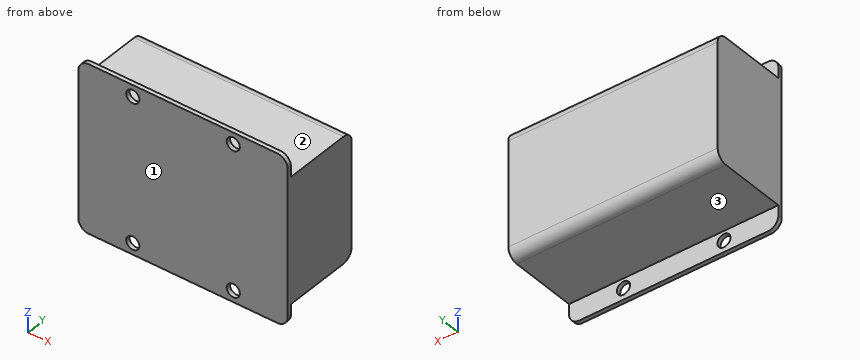
```python
from build123d import *

# Parameters (mm, degrees)
SKETCH_1_W      = 100.2
SKETCH_1_H      = 80
SKETCH_1_R      = 3.14
EXTRUDE_1_DEPTH = 2
SKETCH_3_W      = 100.2
SKETCH_3_H      = 60
EXTRUDE_2_DEPTH = 37
FILLET_1_R      = 5
FILLET_2_R      = 5


with BuildPart() as part:
    # 草图1 → 凸台-拉伸1 (new body)
    with BuildSketch(Plane(origin=(0, 0, 0), x_dir=(1, 0, 0), z_dir=(0, 1, 0))):
        with Locations((0.09, 0)):
            Rectangle(SKETCH_1_W, SKETCH_1_H)
        with Locations(Location((-23.96, 34.55, 0), (0, 0, 270))):
            Circle(SKETCH_1_R, mode=Mode.SUBTRACT)
        with Locations(Location((24.14, 34.55, 0), (0, 0, 270))):
            Circle(SKETCH_1_R, mode=Mode.SUBTRACT)
        with Locations(Location((24.14, -34.55, 0), (0, 0, 270))):
            Circle(SKETCH_1_R, mode=Mode.SUBTRACT)
        with Locations(Location((-23.96, -34.55, 0), (0, 0, 270))):
            Circle(SKETCH_1_R, mode=Mode.SUBTRACT)
    extrude(amount=EXTRUDE_1_DEPTH)

    # 草图3 → 凸台-拉伸2 (add)
    with BuildSketch(Plane(origin=(0, 2, 0), x_dir=(1, 0, 0), z_dir=(0, 1, 0))):
        with Locations((0.09, 0)):
            Rectangle(SKETCH_3_W, SKETCH_3_H)
    extrude(amount=EXTRUDE_2_DEPTH)

    # 圆角1
    fillet_1_edges = [part.edges().sort_by_distance(p)[0] for p in [
        (-50.01, 1, -40),
        (50.19, 1, -40),
        (50.19, 1, 40),
        (-50.01, 1, 40),
    ]]
    fillet(fillet_1_edges, radius=FILLET_1_R)

    # 圆角2
    fillet_2_edges = [part.edges().sort_by_distance(p)[0] for p in [
        (0.09, 39, 30),
        (0.09, 39, -30),
    ]]
    fillet(fillet_2_edges, radius=FILLET_2_R)


solid = part.part
```
Input: part model. Units: mm. Frame: model coordinates. Face numbers are marked on the shaded views. A direction names the side the tool comes from. Coordinates: 2 decimals unless noted, no trailing zeros. Loops run counter-clockwise (first coordinate to the right, second up) from the corner with the lowest first, then second, coordinate; pieces in that order, holes last. Notation, with made-up numbers: M 7.25,-14.5 L 32.25,-14.5 A20 cw 32.25,-9.5 Z; hole C -36,28 d4. An arc over 180 degrees is marked long. Use a Markdown table: item, result. Add a question column.
1) Line query: L1, parallel to X at y = 1.1, z = 34.55; L2, parallel to X at y = 1, z = -34; L3, parallel to Z at x = 3.5, y = 20. Output: solid intervals per line, ascending. Write a range as from..to.
2) Section B-B, the plane x = 43. Return the cut outline in (y, z).
3) Section A-A, the plane x = -23.96. Return the cut outline in (y, z).
4) Pin query (flat end, axial travel): P1, Ø1, axis at x = 7, y = 20, coming from the +Z side; P2, Ø8, axis at x = 24.14, z = 34.55, coming from the -Y side; P3, Ø9.5, axis at x = -19, y = 16, coming from the -Z side; P4, Ø3, axis at x = 19.5, z = -32.5, coming from the +Y side. Return the tip coordinate at first contact, or that it passes through.
5) Set-up query: the marked faces 1, 2 and 3. Return all of +Z, -Z, +X, -X, +Y, -Y with unobstructed straight access to the full face (end or side cutting, diameter ignored); none if empty.
6) Section C-C, the plane y = 11. Return the cut outline in (x, z).
Answer below:
| question | item | result |
|---|---|---|
| 1 | L1 | -50.01..-27.1, -20.82..21, 27.28..50.19 |
| 1 | L2 | -50.01..-27.05, -20.87..21.05, 27.23..50.19 |
| 1 | L3 | -30..30 |
| 2 | outline | M 0,-40 L 2,-40 L 2,-30 L 34,-30 A5 ccw 39,-25 L 39,25 A5 ccw 34,30 L 2,30 L 2,40 L 0,40 Z |
| 3 | outline | M 0,-40 L 2,-40 L 2,-37.69 L 0,-37.69 Z; M 0,-31.41 L 2,-31.41 L 2,-30 L 34,-30 A5 ccw 39,-25 L 39,25 A5 ccw 34,30 L 2,30 L 2,31.41 L 0,31.41 Z; M 0,37.69 L 2,37.69 L 2,40 L 0,40 Z |
| 4 | P1 | z = 30 |
| 4 | P2 | y = 0 |
| 4 | P3 | z = -30 |
| 4 | P4 | y = 2 |
| 5 | face 1 | +Z, -Z, +X, -X, -Y |
| 5 | face 2 | +Z, +X, -X, +Y |
| 5 | face 3 | -Z, +X, -X, +Y |
| 6 | outline | M -50.01,-30 L 50.19,-30 L 50.19,30 L -50.01,30 Z |
